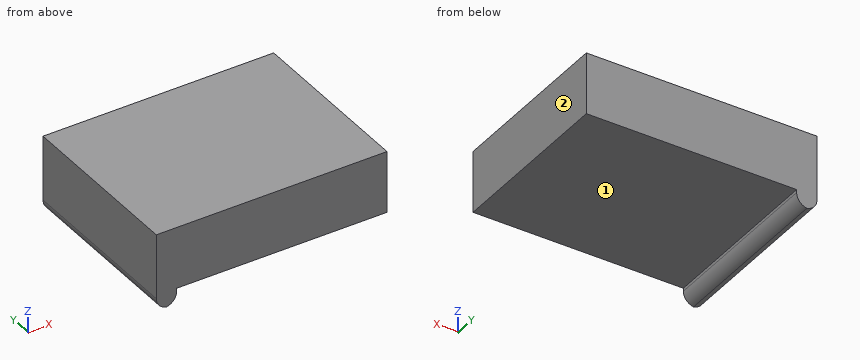
from build123d import *

# Parameters (mm, degrees)
F0_W        = 95.0071103871
F0_H        = 72.4661517888
F1_DEPTH    = 25.4
F2_W        = 8.3860605955
F2_H        = 72.4661517888
F3_DEPTH    = 6.35
F4_T1_DEPTH = 97.8661517888


# Not quite as in the source:
# - a fillet or chamfer that OpenCascade refuses, or shapes differently, is made with other operations: its cross-section is extruded or revolved along the edge and cut away or added


with BuildPart() as f1:
    # F0 (on Top) → F1 (new body)
    with BuildSketch(Plane.XY):
        with Locations((-23.8963868469, 6.1882724985)):
            Rectangle(F0_W, F0_H)
    extrude(amount=F1_DEPTH)

    # F2 (on face) → F3 (join)
    with BuildSketch(Plane(origin=(0, 0, 0), x_dir=(1, 0, 0), z_dir=(0, 0, -1))):
        with Locations((-67.2069117427, -6.1882724985)):
            Rectangle(F2_W, F2_H)
    extrude(amount=F3_DEPTH)

    # F4: fillet of radius 5.08 on 2 edges, made by hand

    # F4_s2 → F4_t1 (cut)
    with BuildSketch(Plane.XZ.offset(-55.121348393)):
        with BuildLine():
            ThreePointArc((-68.0938814449, -6.35), (-64.5017789965, -4.8621024484), (-63.0138814449, -1.27))
            Line((-63.0138814449, -1.27), (-63.0138814449, -6.35))
            Line((-63.0138814449, -6.35), (-68.0938814449, -6.35))
        make_face()
        with BuildLine():
            ThreePointArc((-71.3999420404, -1.27), (-69.9120444889, -4.8621024484), (-66.3199420404, -6.35))
            Line((-66.3199420404, -6.35), (-71.3999420404, -6.35))
            Line((-71.3999420404, -6.35), (-71.3999420404, -1.27))
        make_face()
    extrude(amount=F4_T1_DEPTH, mode=Mode.SUBTRACT)


solid = f1.part
Read the model definition and answer for the solid it produces. Units are mm, in the model's axes. Face numbers are marked on the shaded views. A direction names the side the tool comes from. Coordinates: 2 decimals unless noted, no trailing zeros. Order: outer loops, then holes, each group sorted by start corner. A loop starts at its lowest first (then second) coordinate and runs counter-clockwise, first axis right, second up. Notation, with made-up numbers: (-10, 61.25) -> (38, 61.25) arc R18 ccw to (38, 82.25) -> close; hole circle Ø9 at (19.25, 80). An arc over 180 degrees is marked (long way). Answer as a JSON object with one key per item and string values.
1) This flat-tipped pin is pushed along its axis until it touches: pin 1 (3 mm diameter, centred on x = -44, y = -18.5, fed in from -Z). Where does it stop, or does it pass through?
Model answer:
{"pin 1": "stops at z = 0"}
2) Consider line 1 along Z through (x, y) = (-17, -24); line 2 along Z through (x, y) = (-67, -8.5); line 3 along X through (y, z) = (8, -2). Determine where each line is inside the solid, lowest interval first. Write a range as from..to.
Model answer:
{"line 1": "z = 0..25.4", "line 2": "z = -6.23..25.4", "line 3": "x = -71.35..-63.07"}
3) A cutting plane is placed at B-B, the plane x = -14. Determine the outline of the cut face in (y, z), plus the area to 3 significant figures.
Model answer:
{"outline": "(-30.04, 0) -> (42.42, 0) -> (42.42, 25.4) -> (-30.04, 25.4) -> close", "area": "1,840 mm²"}
4) A cutting plane is placed at A-A, the plane y = -13. Determine the outline of the cut face in (x, z).
Model answer:
{"outline": "(-71.4, -1.27) arc R5.08 ccw to (-67.21, -6.27) arc R5.08 ccw to (-63.01, -1.27) -> (-63.01, 0) -> (23.61, 0) -> (23.61, 25.4) -> (-71.4, 25.4) -> close"}
5) A tool of negligible diameter and unlimited length cuts with its end or side. For the marked faces 1 and 2, from which of +Z, -Z, +X, -X, +Y, -Y can it reach the whole face along a straight path? Write none if from no direction.
Model answer:
{"face 1": "-Z, +X, +Y, -Y", "face 2": "+Z, -Z, +X, +Y, -Y"}
